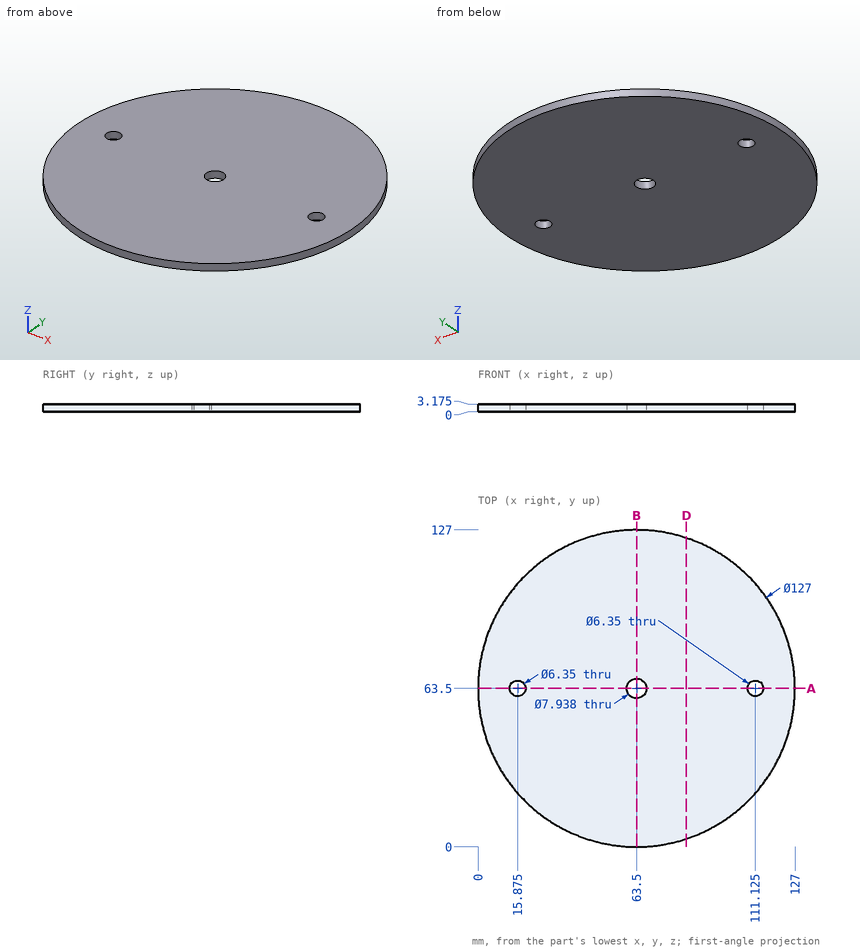
Geometry: see drawing. Coordinates: mm, zero at the bounding-box minimum. Round coordinates to 2 decimals unless told otherwise and drop trailing zeros. Write each loop counter-clockwise with the first axis right and the second up, starting at its lowest first coordinate (ties: lowest second). Pieces come first, ordered by that corner, then holes. Notation, with made-up numbers: (55, 78) - (80, 78) arc R27 ccw to (80, 114) - close; hole circle Ø1 at (75.25, 68.25). An arc over 180 degrees is marked (long way). Use CSV: the item, a comma, the result in double quotes. Start each with the question number.
(1) Cut plane B-B, the plane x = 63.5. Return loops of the section in (y, z) (1 decimal).
(2) Cut plane D-D, the plane x = 83.5. Return loops of the section in (y, z) (1 decimal).
(3) Material intervals for probe 1 along Y at (x, z) = (63.5, 1.1); probe 2 along X at (y, z) = (64, 2.15); probe 3 along Y at (x, z) = (14.5, 1.5) (1 decimal), sorted ascending. Write a range as [from, to].
(4) First-contact query: pin 1 Ø1.5 at (y, z) = (51, 0.5) entering from +X. Flat tip, straight axial feed; report the tip coordinate or a pass-through.
(5) Cut plane A-A, the plane y = 63.5. Give the number of separate pieces and of enclosed holes in the cut face.
Geometry says:
1,outline,"(0, 0) - (59.5, 0) - (59.5, 3.2) - (0, 3.2) - close; (67.5, 0) - (127, 0) - (127, 3.2) - (67.5, 3.2) - close"
2,outline,"(3.2, 0) - (123.8, 0) - (123.8, 3.2) - (3.2, 3.2) - close"
3,probe 1,"[0, 59.53], [67.47, 127]"
3,probe 2,"[0, 12.74], [19.01, 59.56], [67.44, 107.99], [114.26, 127]"
3,probe 3,"[23.1, 60.6], [66.4, 103.9]"
4,pin 1,"x = 125.9"
5,separate pieces,"4"
5,enclosed holes,"0"
